Could you check a few things on this model? Use its own coordinates, in mm. Face numbers are marked on the shaded views. A direction names the side the tool comes from. Round coordinates to 2 decimals unless told otherwise and drop trailing zeros. Loops run counter-clockwise (first coordinate to the right, second up) from the corner with the lowest first, then second, coordinate; pieces in that order, holes last. Notation, with made-up numbers: (37.25, 64) -> (95.25, 64) arc R29 cw to (95.25, 97) -> close; hole circle Ø9 at (40, 62). An arc over 180 degrees is marked (long way). Put each result on its own line as item: value. Start each with the question number.
1. I need wall thicknesses on line 1 (Y direction, x = 39.5, z = 7); line 2 (X direction, y = -14, z = 2.5); line 3 (Z direction, x = 7, y = -25.5). Which ranges of each line are inside material? Lowest first, please. Write a range as [from, to].
2. If we mould it in two halves opening along Y, with no side actions, what happens to the marked faces 1, 2, 3 and 4? For each: pulls with the +Y half, pulls with the -Y half, needs draft (parallel to the pull), parting line crosses it, or undercut.
3. Imagine slicing it at B-B, the plane z = 4. Please give me the cut outline in (x, y).
4. Imagine slicing it at A-A, the plane z = 0. Count the separate pieces of the cut face and the enclosed holes in it, and give its area (3 significant figures).
5. Imagine slicing it at D-D, the plane y = -27.5. Please give me the cut outline in (x, z), and give its area (3 significant figures).
6. Imagine slicing it at C-C, the plane x = -18. Please give me the cut outline in (y, z), and give its area (3 significant figures).
7. Which directions (+Z, -Z, +X, -X, +Y, -Y) give clear straight access to the entire face, cutting with the end or side of a thin tool? Please do the marked faces 5 and 6.
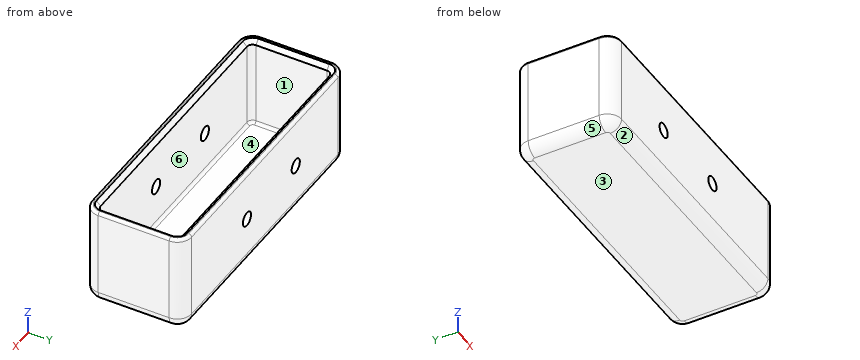
```python
from build123d import *

# Parameters (mm, degrees)
F0_W     = 100
F0_H     = 35
F1_DEPTH = 35
F2_R     = 5
F3_R     = 4
F4_T     = -3
F6_D     = 5
F7_SIZE  = 1.5
F8_R     = 1


with BuildPart() as f1:
    # F0 (on Front) → F1 (new body)
    with BuildSketch(Plane.XZ):
        Rectangle(F0_W, F0_H)
    extrude(amount=F1_DEPTH)

    # F2
    f2_edges = [f1.edges().sort_by_distance(p)[0] for p in [
        (50, -35, 0),
        (50, 0, 0),
        (-50, -35, 0),
        (-50, 0, 0),
    ]]
    fillet(f2_edges, radius=F2_R)

    # F3
    f3_edges = [f1.edges().sort_by_distance(p)[0] for p in [
        (0, -35, -17.5),
    ]]
    fillet(f3_edges, radius=F3_R)

    # F4
    f4_openings = [f1.faces().sort_by_distance(p)[0] for p in [
        (0, -17.5, 17.5),
    ]]
    offset(amount=F4_T, openings=f4_openings)

    # F6 (through all)
    with Locations(Plane.XZ.offset(35)):
        with Locations((-19.0995354205, 0), (10.9004645795, 0)):
            Hole(F6_D / 2)

    # F7
    f7_edges = [f1.edges().sort_by_distance(p)[0] for p in [
        (-47, -17.5, 17.5),
        (0, -3, 17.5),
        (47, -17.5, 17.5),
        (0, -32, 17.5),
    ]]
    chamfer(f7_edges, length=F7_SIZE)

    # F8
    f8_edges = [f1.edges().sort_by_distance(p)[0] for p in [
        (-50, -17.5, 17.5),
    ]]
    fillet(f8_edges, radius=F8_R)


solid = f1.part
```
Entries:
1. line 1: [-35, -32], [-3, 0]
1. line 2: [-50, -47], [47, 50]
1. line 3: [-17.5, -14.5]
2. face 1: undercut
2. face 2: pulls with the -Y half
2. face 3: needs draft
2. face 4: undercut
3. outline: (-50, -30) arc R5 ccw to (-45, -35) -> (45, -35) arc R5 ccw to (50, -30) -> (50, -5) arc R5 ccw to (45, 0) -> (-45, 0) arc R5 ccw to (-50, -5) -> close; hole (-47, -30) arc R2 ccw to (-45, -32) -> (45, -32) arc R2 ccw to (47, -30) -> (47, -5) arc R2 ccw to (45, -3) -> (-45, -3) arc R2 ccw to (-47, -5) -> close
4. separate pieces: 4
4. enclosed holes: 0
4. area: 696 mm^2
5. outline: (-50, -13.5) arc R4 ccw to (-46, -17.5) -> (46, -17.5) arc R4 ccw to (50, -13.5) -> (50, 16.5) arc R1 ccw to (49, 17.5) -> (48.5, 17.5) -> (47, 16) -> (47, -13.5) arc R1 cw to (46, -14.5) -> (-46, -14.5) arc R1 cw to (-47, -13.5) -> (-47, 16) -> (-48.5, 17.5) -> (-49, 17.5) arc R1 ccw to (-50, 16.5) -> close
5. area: 483 mm^2
6. outline: (-35, -13.5) arc R4 ccw to (-31, -17.5) -> (-4, -17.5) arc R4 ccw to (0, -13.5) -> (0, -2.25) -> (-3, -2.25) -> (-3, -13.5) arc R1 cw to (-4, -14.5) -> (-31, -14.5) arc R1 cw to (-32, -13.5) -> (-32, -2.25) -> (-35, -2.25) -> close; (-35, 2.25) -> (-32, 2.25) -> (-32, 16) -> (-33.5, 17.5) -> (-34, 17.5) arc R1 ccw to (-35, 16.5) -> close; (-3, 2.25) -> (0, 2.25) -> (0, 16.5) arc R1 ccw to (-1, 17.5) -> (-1.5, 17.5) -> (-3, 16) -> close
6. area: 261 mm^2
7. face 5: -Z, -X, +Y, -Y
7. face 6: +Z
